```python
from build123d import *

# Parameters (mm, degrees)
CIRCLE_R           = 4.26
EXTRUSION001_DEPTH = 34.920666
RECTANGLE_W        = 28.2
RECTANGLE_H        = 58
EXTRUSION_DEPTH    = 2


with BuildPart() as extrusion001:
    # Circle → Extrusion001 (new body)
    with BuildSketch(Plane(origin=(-279.976256, -51.600832, -5.133948), x_dir=(0, 1, 0), z_dir=(0, 0, -1))):
        Circle(CIRCLE_R)
    extrude(amount=-EXTRUSION001_DEPTH)


with BuildPart() as cut001:
    # Rectangle → Extrusion (new body)
    with BuildSketch(Plane(origin=(-309.476256, -65.700832, -5.133948), x_dir=(0, 1, 0), z_dir=(0, 0, -1))):
        with Locations((14.1, 29)):
            Rectangle(RECTANGLE_W, RECTANGLE_H)
    extrude(amount=-EXTRUSION_DEPTH)

    # Cut001: cut Extrusion001
    add(extrusion001.part, mode=Mode.SUBTRACT)


solid = cut001.part
```
Read the model definition and answer for the solid it produces. Units are mm, in the model's axes. Coordinates: 2 decimals unless noted, no trailing zeros. Order: outer loops, then holes, each group sorted by start corner. A loop starts at its lowest first (then second) coordinate and runs counter-clockwise, first axis right, second up. Notation, with made-up numbers: (59.5, 31.5) - (80.5, 31.5) arc R33 ccw to (80.5, 66.5) - close; hole circle Ø11 at (42.5, 53.5). An arc over 180 degrees is marked (long way). Answer as a JSON object with one key per item and string values. Group by question number.
Item 1: Section C-C (z = -4.3) is taken. Give the vertices of the cut face in (x, y).
Item 2: A flat-ended cylindrical pin translates along its axis: P1, Ø11, axis at x = -279.98, y = -51.6, coming from the +Z side. Find the tip coordinate at first contact, or state that the pin passes through.
Item 3: Section B-B (y = -53.5) is taken. Give the vertices of the cut face in (x, z), plus the area to 3 significant figures.
Item 4: Section A-A (x = -277) is taken. Give the vertices of the cut face in (y, z), plus the area to 3 significant figures.
Item 5: The mould has two halves that part along X. Classify faces 1 (the face through (-280, -58, -3.134)), 2 (the face through (-284, -53, -4)), 3 (the face through (-309.476, -52, -4)), 4 (the face through (-251.476, -52, -4)): +X half, -X half, draft (parallel to the pull), parting line (faces both ways), or undercut.
Item 6: Consider probe 1 along X at (y, z) = (-51.75, -3.55); probe 2 along Y at (x, z) = (-278, -4.75); probe 3 along X at (y, z) = (-48, -4.3). Determine where each line is inside the solid, lowest interval first. Write a range as from..to.
Results are:
{
 "1": {"outline": "(-309.48, -65.7) - (-251.48, -65.7) - (-251.48, -37.5) - (-309.48, -37.5) - close; hole circle Ø8.52 at (-279.98, -51.6)"},
 "2": {"P1": "stops at z = -3.13"},
 "3": {"outline": "(-309.48, -5.13) - (-283.79, -5.13) - (-283.79, -3.13) - (-309.48, -3.13) - close; (-276.16, -5.13) - (-251.48, -5.13) - (-251.48, -3.13) - (-276.16, -3.13) - close", "area": "101 mm^2"},
 "4": {"outline": "(-65.7, -5.13) - (-54.65, -5.13) - (-54.65, -3.13) - (-65.7, -3.13) - close; (-48.55, -5.13) - (-37.5, -5.13) - (-37.5, -3.13) - (-48.55, -3.13) - close", "area": "44.2 mm^2"},
 "5": {"face 1": "draft", "face 2": "undercut", "face 3": "-X half", "face 4": "+X half"},
 "6": {"probe 1": "x = -309.48..-284.23, -275.72..-251.48", "probe 2": "y = -65.7..-55.37, -47.83..-37.5", "probe 3": "x = -309.48..-282.25, -277.7..-251.48"}
}
